Verification items for the finished model (mm, model axes). Round coordinates to 2 decimals unless told otherwise and drop trailing zeros. Order: outer loops, then holes, each group sorted by start corner. A loop starts at its lowest first (then second) coordinate and runs counter-clockwise, first axis right, second up.
```python
from build123d import *

# Parameters (mm, degrees)
SKETCH2_R           = 1.475
SKETCH2_R_2         = 36.5
SKETCH2_W           = 19.05
SKETCH2_H           = 25.4
SKETCH2_H_2         = 7.933333334
BOSS_EXTRUDE1_DEPTH = 0.508
FILLET1_R           = 6.35


with BuildPart() as part:
    # Sketch2 → Boss-Extrude1 (new body)
    # profile 1 of 7: a face of its own
    with BuildSketch(Plane.XY):
        Polygon((57.15, 50), (-57.15, 50), (-57.15, 29.366666667), (-57.15, 3.966666667), (-57.15, -3.966666667), (-57.15, -18.966666667), (0, -45), (57.15, -18.966666667), (57.15, -3.966666667), (57.15, 3.966666667), (57.15, 29.366666667), align=None)
        with Locations((-50.8, 0)):
            Circle(SKETCH2_R, mode=Mode.SUBTRACT)
        Circle(SKETCH2_R_2, mode=Mode.SUBTRACT)
        with Locations((50.8, 0)):
            Circle(SKETCH2_R, mode=Mode.SUBTRACT)
    # profile 2 of 7: a face of its own
    with BuildSketch(Plane.XY):
        with Locations((-66.675, 16.666666667)):
            Rectangle(SKETCH2_W, SKETCH2_H)
    # profile 3 of 7: a face of its own
    with BuildSketch(Plane.XY):
        with Locations((-66.675, 0)):
            Rectangle(SKETCH2_W, SKETCH2_H_2)
        with Locations((-63.5, 0)):
            Circle(SKETCH2_R, mode=Mode.SUBTRACT)
    # profile 4 of 7: a face of its own
    with BuildSketch(Plane.XY):
        Polygon((-57.15, -18.966666667), (-57.15, -3.966666667), (-76.2, -3.966666667), (-76.2, -10.288888889), align=None)
    # profile 5 of 7: a face of its own
    with BuildSketch(Plane.XY):
        Polygon((76.2, -3.966666667), (57.15, -3.966666667), (57.15, -18.966666667), (76.2, -10.288888889), align=None)
    # profile 6 of 7: a face of its own
    with BuildSketch(Plane.XY):
        with Locations((66.675, 0)):
            Rectangle(SKETCH2_W, SKETCH2_H_2)
        with Locations((63.5, 0)):
            Circle(SKETCH2_R, mode=Mode.SUBTRACT)
    # profile 7 of 7: a face of its own
    with BuildSketch(Plane.XY):
        with Locations((66.675, 16.666666667)):
            Rectangle(SKETCH2_W, SKETCH2_H)
    extrude(amount=BOSS_EXTRUDE1_DEPTH)

    # Fillet1
    fillet1_edges = [part.edges().sort_by_distance(p)[0] for p in [
        (0, -45, 0.254),
        (-76.2, -10.288888889, 0.254),
        (-76.2, 29.366666667, 0.254),
        (-57.15, 50, 0.254),
        (57.15, 50, 0.254),
        (76.2, 29.366666667, 0.254),
        (76.2, -10.288888889, 0.254),
    ]]
    fillet(fillet1_edges, radius=FILLET1_R)


solid = part.part
```
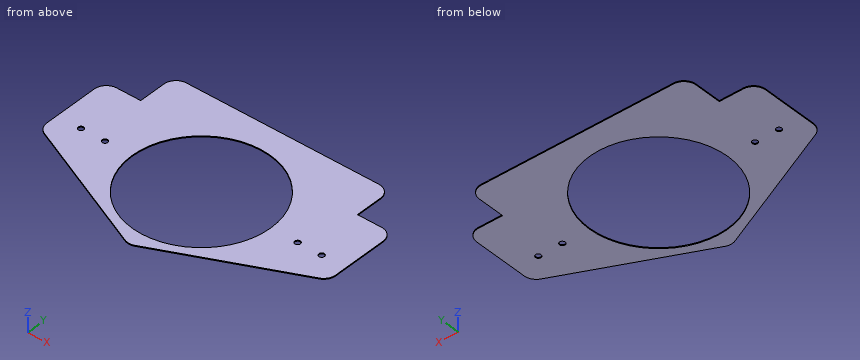
1) Sectioned sample at B-B on y = 0. Record the cut outline in (x, z) (3 decimals), then the cut area to 3 significant figures.
2) Sectioned sample at A-A on x = 0. Record the cut outline in (y, z).
3) Sectioned sample at D-D on y = 19.5. Record the cut outline in (x, z).
4) Sectioned sample at C-C on z = 0.25. Record the cut outline in (x, y) (3 decimals).
5) Scan lines: probe 1 along Y at (x, z) = (0, 0.1); probe 2 along X at (y, z) = (14, 0.35); probe 3 along X at (y, z) = (3.5, 0.25). Record each from-to range of solid material in increasing order.
Returned:
1. outline: (-76.2, 0) - (-64.975, 0) - (-64.975, 0.508) - (-76.2, 0.508) - close; (-62.025, 0) - (-52.275, 0) - (-52.275, 0.508) - (-62.025, 0.508) - close; (-49.325, 0) - (-36.5, 0) - (-36.5, 0.508) - (-49.325, 0.508) - close; (36.5, 0) - (49.325, 0) - (49.325, 0.508) - (36.5, 0.508) - close; (52.275, 0) - (62.025, 0) - (62.025, 0.508) - (52.275, 0.508) - close; (64.975, 0) - (76.2, 0) - (76.2, 0.508) - (64.975, 0.508) - close
1. area: 34.3 mm2
2. outline: (-44.37, 0) - (-36.5, 0) - (-36.5, 0.51) - (-44.37, 0.51) - close; (36.5, 0) - (50, 0) - (50, 0.51) - (36.5, 0.51) - close
3. outline: (-76.2, 0) - (-30.85, 0) - (-30.85, 0.51) - (-76.2, 0.51) - close; (30.85, 0) - (76.2, 0) - (76.2, 0.51) - (30.85, 0.51) - close
4. outline: (-76.2, -6.204) arc R6.35 ccw to (-72.482, -11.982) - (-2.632, -43.801) arc R6.35 ccw to (2.632, -43.801) - (72.482, -11.982) arc R6.35 ccw to (76.2, -6.204) - (76.2, 23.017) arc R6.35 ccw to (69.85, 29.367) - (57.15, 29.367) - (57.15, 43.65) arc R6.35 ccw to (50.8, 50) - (-50.8, 50) arc R6.35 ccw to (-57.15, 43.65) - (-57.15, 29.367) - (-69.85, 29.367) arc R6.35 ccw to (-76.2, 23.017) - close; hole circle Ø2.95 at (-63.5, 0); hole circle Ø2.95 at (-50.8, 0); hole circle Ø73 at (0, 0); hole circle Ø2.95 at (50.8, 0); hole circle Ø2.95 at (63.5, 0)
5. probe 1: y = -44.37 to -36.5, 36.5 to 50
5. probe 2: x = -76.2 to -33.71, 33.71 to 76.2
5. probe 3: x = -76.2 to -36.33, 36.33 to 76.2
